Autodesk Inventor part; units mm, degrees
ref_plane "YZ Plane" through (0, 0, 0) normal (1, 0, 0) x (0, 1, 0)
ref_plane "XZ Plane" through (0, 0, 0) normal (0, 1, 0) x (-1, 0, 0)
ref_plane "XY Plane" through (0, 0, 0) normal (0, 0, 1) x (1, 0, 0)
sketch "Sketch1" plane through (0, 0, 0) normal (0, 0, 1) x (1, 0, 0)
  line L0 (-62.5, 65.8108) -> (62.5, 65.8108)
  line L1 (62.5, 65.8108) -> (62.5, -64.1892)
  line L2 (62.5, -64.1892) -> (-62.5, -64.1892)
  line L3 (-62.5, -64.1892) -> (-62.5, 65.8108)
  line L4 (-47.5, -9.1892) -> (47.5, -9.1892)
  line L5 (47.5, -9.1892) -> (47.5, -49.1892)
  line L6 (47.5, -49.1892) -> (-47.5, -49.1892)
  line L7 (-47.5, -49.1892) -> (-47.5, -9.1892)
  line L8 (-62.5, 5.8108) -> (62.5, 5.8108)
  point P0 (0, 0)
  point P1 (-50, 18)
  point P2 (50, 18)
  point P3 (0, 18)
  dimension "d0" = 125
  dimension "d1" = 62.5
  dimension "d2" = 60
  dimension "d3" = 15
  dimension "d4" = 40
  dimension "d5" = 15
  dimension "d6" = 15
  dimension "d7" = 15
  dimension "d8" = 100
  dimension "d9" = 12.5
  dimension "d24" = 50
extrude "Extrusion1" add sketch "Sketch1" along normal blind 6
hole "Hole1" at (-50, 18, 0) at (50, 18, 0) at (0, 18, 0) direction (0, 0, 1) diameter 3.5 end through all
chamfer "Chamfer1" distance 40 angle 45 2 edges at (-62.5, 65.8108, 3) (62.5, 65.8108, 3)
fillet "Fillet1" radius 5 6 edges at (47.5, -9.1892, 3) (47.5, -49.1892, 3) (62.5, -64.1892, 3) (-62.5, -64.1892, 3) (-47.5, -49.1892, 3) (-47.5, -9.1892, 3)
fillet "Fillet2" radius 5 4 edges at (-62.5, 25.8108, 3) (-22.5, 65.8108, 3) (22.5, 65.8108, 3) (62.5, 25.8108, 3)
sketch "Sketch2" plane through (0, 0, 6) normal (0, 0, 1) x (1, 0, 0)
  circle A0 centre (0, 18) radius 1.75
  circle A1 centre (50, 18) radius 1.75
  circle A2 centre (-50, 18) radius 1.75
  arc A3 (62.5, 23.7397) -> (61.0355, 27.2753) centre (57.5, 23.7397) ccw
  line L0 (23.9645, 64.3463) -> (61.0355, 27.2753)
  arc A4 (23.9645, 64.3463) -> (20.4289, 65.8108) centre (20.4289, 60.8108) ccw
  line L1 (20.4289, 65.8108) -> (-20.4289, 65.8108)
  arc A5 (-20.4289, 65.8108) -> (-23.9645, 64.3463) centre (-20.4289, 60.8108) ccw
  line L2 (-61.0355, 27.2753) -> (-23.9645, 64.3463)
  arc A6 (-61.0355, 27.2753) -> (-62.5, 23.7397) centre (-57.5, 23.7397) ccw
  line L3 (-62.5, 23.7397) -> (-62.5, -59.1892)
  arc A7 (-62.5, -59.1892) -> (-57.5, -64.1892) centre (-57.5, -59.1892) ccw
  line L4 (-57.5, -64.1892) -> (57.5, -64.1892)
  arc A8 (57.5, -64.1892) -> (62.5, -59.1892) centre (57.5, -59.1892) ccw
  line L5 (62.5, -59.1892) -> (62.5, 23.7397)
  line L6 (-42.5, -9.1892) -> (42.5, -9.1892)
  arc A9 (47.5, -14.1892) -> (42.5, -9.1892) centre (42.5, -14.1892) ccw
  line L7 (47.5, -14.1892) -> (47.5, -44.1892)
  arc A10 (42.5, -49.1892) -> (47.5, -44.1892) centre (42.5, -44.1892) ccw
  line L8 (42.5, -49.1892) -> (-42.5, -49.1892)
  arc A11 (-47.5, -44.1892) -> (-42.5, -49.1892) centre (-42.5, -44.1892) ccw
  line L9 (-47.5, -44.1892) -> (-47.5, -14.1892)
  arc A12 (-42.5, -9.1892) -> (-47.5, -14.1892) centre (-42.5, -14.1892) ccw
  point P0 (0, 0)
  point P1 (16, 53)
  point P2 (-16, 53)
  dimension "d25" = 16
  dimension "d26" = 16
  dimension "d27" = 35
hole "Hole2" at (16, 53, 6) at (-16, 53, 6) direction (0, 0, -1) diameter 3.5 end through all
equation "\"d5\" = d3"
equation "\"d6\" = d3"
equation "\"d7\" = d5"
properties part number "3DP_PLA_Handle"
Model file for the job. Use its own axes, mm. A direction names the side the tool comes from. Coordinates: 2 decimals unless noted, no trailing zeros. Write each loop counter-clockwise with the first axis right and the second up, starting at its lowest first coordinate (ties: lowest second). Pieces come first, ordered by that corner, then holes. Notation, with made-up numbers: (4, 1.25) - (40, 1.25) arc R13 ccw to (40, 8.25) - close; hole circle Ø2 at (16, 7). An arc over 180 degrees is marked (long way). One line per item, written item: value. Start each with the question number.
1. Slice it at B-B (x = 0). Write the cut outline in (y, z).
2. Probe line 1 (X direction, y = 18, z = 2.85); line 2 (Y direction, x = 0, z = 2.5); line 3 (Y direction, x = -19.5, z = 1.85). List the from-to ranges inside material, lowest first. Write a range as from..to.
3. Slice it at D-D (y = 53). Write the cut outline in (x, z).
4. Slice it at A-A (y = -36.5). Write the cut outline in (x, z).
5. Slice it at C-C (z = 2.55). Write the cut outline in (x, y), plus the area to 3 significant figures.
6. Mould opens along X. For faces 1 (the flat face through (1, -64.189, 3)), 2 (the cylindrical face through (46, -47.76, 3.04)), 3 (the flat face through (-42.76, 45.55, 3.04)) say: released by +X, released by -X, zero draft, split by the parting line, or undercut.
7. Tool access for faces 4 (the cylindrical face through (61, -62.76, 3.04)), 5 (the cylindrical face through (-46, -10.62, 3.04)): list every direction of +Z, -Z, +X, -X, +Y, -Y with a clear straight run to the whole face (end or side of a thin tool).
Answers below:
1. outline: (-64.19, 0) - (-49.19, 0) - (-49.19, 6) - (-64.19, 6) - close; (-9.19, 0) - (16.25, 0) - (16.25, 6) - (-9.19, 6) - close; (19.75, 0) - (65.81, 0) - (65.81, 6) - (19.75, 6) - close
2. line 1: x = -62.5..-51.75, -48.25..-1.75, 1.75..48.25, 51.75..62.5
2. line 2: y = -64.19..-49.19, -9.19..16.25, 19.75..65.81
2. line 3: y = -64.19..-49.19, -9.19..65.81
3. outline: (-35.31, 0) - (-17.75, 0) - (-17.75, 6) - (-35.31, 6) - close; (-14.25, 0) - (14.25, 0) - (14.25, 6) - (-14.25, 6) - close; (17.75, 0) - (35.31, 0) - (35.31, 6) - (17.75, 6) - close
4. outline: (-62.5, 0) - (-47.5, 0) - (-47.5, 6) - (-62.5, 6) - close; (47.5, 0) - (62.5, 0) - (62.5, 6) - (47.5, 6) - close
5. outline: (-62.5, -59.19) arc R5 ccw to (-57.5, -64.19) - (57.5, -64.19) arc R5 ccw to (62.5, -59.19) - (62.5, 23.74) arc R5 ccw to (61.04, 27.28) - (23.96, 64.35) arc R5 ccw to (20.43, 65.81) - (-20.43, 65.81) arc R5 ccw to (-23.96, 64.35) - (-61.04, 27.28) arc R5 ccw to (-62.5, 23.74) - close; hole circle Ø3.5 at (-50, 18); hole (-47.5, -44.19) arc R5 ccw to (-42.5, -49.19) - (42.5, -49.19) arc R5 ccw to (47.5, -44.19) - (47.5, -14.19) arc R5 ccw to (42.5, -9.19) - (-42.5, -9.19) arc R5 ccw to (-47.5, -14.19) - close; hole circle Ø3.5 at (-16, 53); hole circle Ø3.5 at (0, 18); hole circle Ø3.5 at (16, 53); hole circle Ø3.5 at (50, 18)
5. area: 10,800 mm^2
6. face 1: zero draft
6. face 2: undercut
6. face 3: released by -X
7. face 4: +Z, -Z, +X, -Y
7. face 5: +Z, -Z
